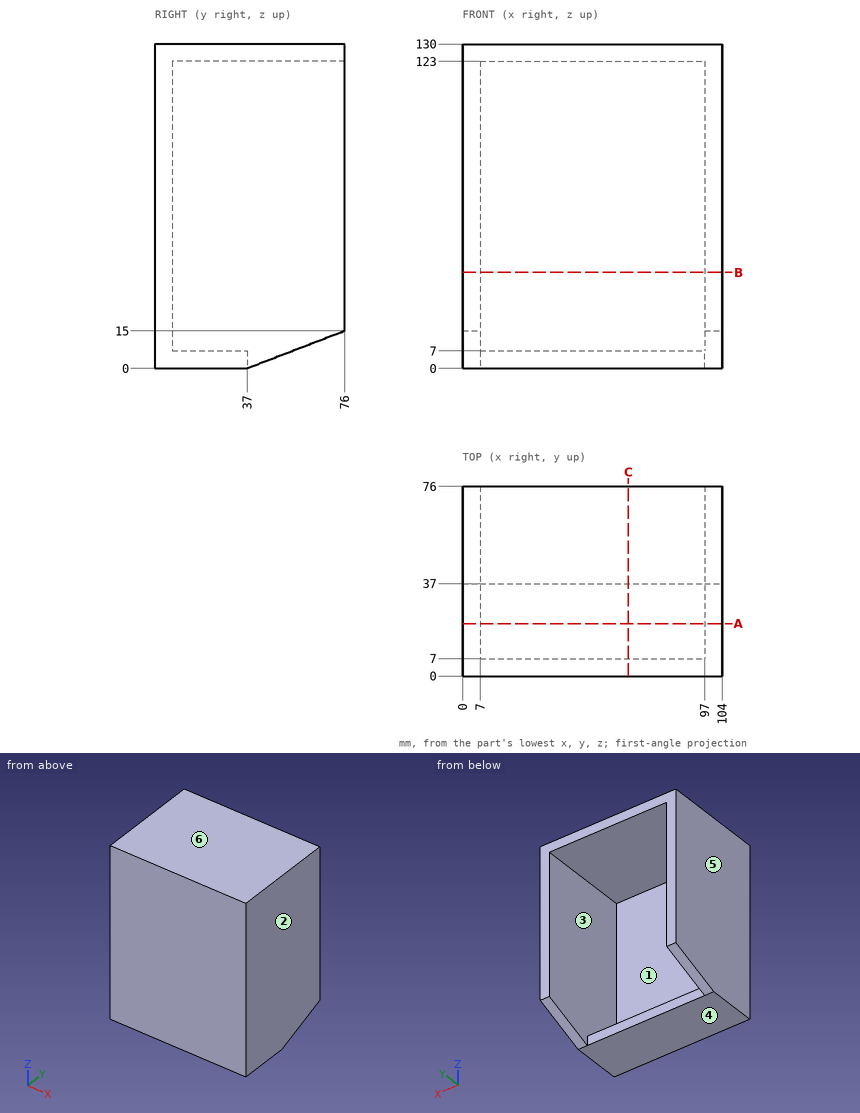
Answer from the drawing. Dimensions are ordinates in mm from the lowest x, y and z of the part. A direction names the side the tool comes from. Round coordinates to 2 decimals unless told otherwise and drop trailing zeros. Loops run counter-clockwise (first coordinate to the right, second up) from the corner with the lowest first, then second, coordinate; pieces in that order, holes last. Notation, with made-up numbers: (85.5, 11) - (130.5, 11) arc R7 cw to (130.5, 16) - close; hole circle Ø10 at (63, -24.75). An arc over 180 degrees is marked (long way). One line per item, written item: value.
Q1. Straight lines are drawn through the part: probe 1 along Z at (x, y) = (51, 23.5); probe 2 along X at (y, z) = (14.5, 22); probe 3 along Y at (x, z) = (41.5, 36.5). For each, find the intervals that lie inside material, in ascending order.
Check values:
probe 1: 0 to 7, 123 to 130
probe 2: 0 to 7, 97 to 104
probe 3: 0 to 7
Q2. Each of these flat-tipped pins is pushed along its axis until it touches: pin 1 Ø8 at (x, y) = (19.5, 60) entering from -Z; pin 2 Ø3.5 at (x, z) = (47.5, 2) entering from +Y. Where does it stop, or does it pass through?
Check values:
pin 1: z = 123
pin 2: y = 37
Q3. Find section A-A on y = 21. Give the vertices of the cut face in (x, z).
Check values:
outline: (0, 0) - (104, 0) - (104, 130) - (0, 130) - close; hole (7, 7) - (97, 7) - (97, 123) - (7, 123) - close
Q4. The mould has two halves that part along Z. Classify the marked faces 3, 4, 5 and 6: +Z half, -Z half, draft (parallel to the pull), parting line (faces both ways), or undercut.
Check values:
face 3: undercut
face 4: -Z half
face 5: draft
face 6: +Z half
Q5. For the marked faces 1 and 2, determine the directions among +Z, -Z, +X, -X, +Y, -Y from which every point of the face is accessible in a straight line to the end or side of a thin tool.
Check values:
face 1: +Y
face 2: +Z, -Z, +X, +Y, -Y
Q6. Find section B-B on z = 38.5. Give the vertices of the cut face in (x, y), and give its area (3 significant figures).
Check values:
outline: (0, 0) - (104, 0) - (104, 76) - (97, 76) - (97, 7) - (7, 7) - (7, 76) - (0, 76) - close
area: 1,690 mm2
Q7. Find section C-C on x = 66.5. Give the vertices of the cut face in (y, z).
Check values:
outline: (0, 0) - (37, 0) - (37, 7) - (7, 7) - (7, 123) - (76, 123) - (76, 130) - (0, 130) - close
